Source: CAD feature listing. Evaluate the final solid. Frame: model axes, mm. Face numbers are marked on the shaded views. Give positions to 0.01 mm unless a question says otherwise; leave off trailing zeros. Order: outer loops, then holes, each group sorted by start corner. A loop starts at its lowest first (then second) coordinate and runs counter-clockwise, first axis right, second up. Notation, with made-up numbers: (37, 80) - (73, 80) arc R14 ccw to (73, 95) - close; hole circle Ø1 at (-24.5, -28). An arc over 180 degrees is marked (long way). Write each question's results on one line, items separated by ' | '. Start each with the question number.
Item 1: Section B-B on z = -22. Output: boundary loops of the cut face in (x, y), and give its area (3 significant figures).
Item 2: Section A-A on x = 11. Output: boundary loops of the cut face in (y, z).
Item 3: Line query: line 1 along X through (y, z) = (-24.2, -3.25); line 2 along X through (y, z) = (-24.7, -34); line 3 along Y through (x, z) = (-8.5, -22). Output: solid intervals per line, ascending.
Item 4: Mould query, pull axis X, two halves, no side actions, for the marked faces 1 and 2. Classes: released by +X, released by -X, zero draft, split by the parting line, or undercut.
Item 5: Contact query for a flat-ended pin moving along its axis: pin 1 Ø3 at (x, z) = (11, -22) entering from -Y. Output: stop coordinate, or through.
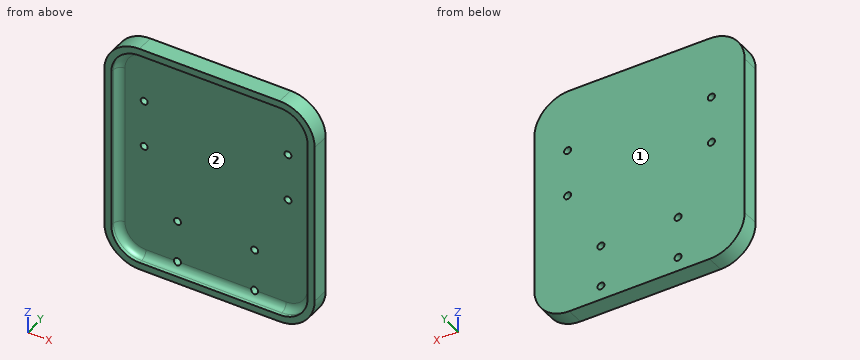
```python
from build123d import *

# Parameters (mm, degrees)
SKETCH1_W           = 60
SKETCH1_H           = 66
BOSS_EXTRUDE1_DEPTH = 5
FILLET1_R           = 10
SHELL1_T            = -2
FILLET2_R           = 2
SKETCH3_R           = 1
CUT_EXTRUDE1_DEPTH  = 5


with BuildPart() as part:
    # Sketch1 → Boss-Extrude1 (new body)
    with BuildSketch(Plane.XZ.offset(23)):
        with Locations((0, -5)):
            Rectangle(SKETCH1_W, SKETCH1_H)
    extrude(amount=BOSS_EXTRUDE1_DEPTH)

    # Fillet1
    fillet1_edges = [part.edges().sort_by_distance(p)[0] for p in [
        (-30, -25.5, 28),
        (30, -25.5, 28),
        (30, -25.5, -38),
        (-30, -25.5, -38),
    ]]
    fillet(fillet1_edges, radius=FILLET1_R)

    # Shell1
    shell1_openings = [part.faces().sort_by_distance(p)[0] for p in [
        (0, -28, -5),
    ]]
    offset(amount=SHELL1_T, openings=shell1_openings, kind=Kind.INTERSECTION)

    # Fillet2
    fillet2_edges = [part.edges().sort_by_distance(p)[0] for p in [
        (-28, -25, -5),
        (0, -25, -36),
        (28, -25, -5),
        (0, -25, 26),
        (25.656854249, -25, -33.656854249),
        (-25.656854249, -25, -33.656854249),
        (-25.656854249, -25, 23.656854249),
        (25.656854249, -25, 23.656854249),
    ]]
    fillet(fillet2_edges, radius=FILLET2_R)

    # Sketch3 → Cut-Extrude1 (cut)
    with BuildSketch(Plane(origin=(0, -23, 0), x_dir=(1, 0, 0), z_dir=(0, 1, 0))):
        with Locations(Location((20.5, 3.25, 0), (0, 0, 270))):
            Circle(SKETCH3_R)
        with Locations(Location((20.5, -10.25, 0), (0, 0, 270))):
            Circle(SKETCH3_R)
        with Locations(Location((11, 34, 0), (0, 0, 270))):
            Circle(SKETCH3_R)
        with Locations(Location((11, 22, 0), (0, 0, 270))):
            Circle(SKETCH3_R)
        with Locations(Location((-11, 34, 0), (0, 0, 270))):
            Circle(SKETCH3_R)
        with Locations(Location((-11, 22, 0), (0, 0, 270))):
            Circle(SKETCH3_R)
        with Locations(Location((-20.5, 3.25, 0), (0, 0, 270))):
            Circle(SKETCH3_R)
        with Locations(Location((-20.5, -10.25, 0), (0, 0, 270))):
            Circle(SKETCH3_R)
    extrude(amount=-CUT_EXTRUDE1_DEPTH, mode=Mode.SUBTRACT)


solid = part.part
```
Evaluation:
1) outline: (-30, -28) - (-28, -28) - (-28, -27) arc R2 cw to (-26, -25) - (-12, -25) - (-12, -23) - (-30, -23) - close; (-10, -25) - (10, -25) - (10, -23) - (-10, -23) - close; (12, -25) - (26, -25) arc R2 cw to (28, -27) - (28, -28) - (30, -28) - (30, -23) - (12, -23) - close | area: 126 mm^2
2) outline: (-28, -38) - (-23, -38) - (-23, -35) - (-25.27, -35) arc R2 cw to (-27, -36) - (-28, -36) - close; (-28, 26) - (-27, 26) arc R2 cw to (-25, 24) - (-25, -21) - (-23, -21) - (-23, 28) - (-28, 28) - close; (-25, -33) - (-23, -33) - (-23, -23) - (-25, -23) - close
3) line 1: x = -30 to -21.5, -19.5 to 19.5, 21.5 to 30 | line 2: x = -28 to -12, -10 to 10, 12 to 28 | line 3: y = -25 to -23
4) face 1: zero draft | face 2: undercut
5) pin 1: stops at y = -25
